from build123d import *

# Parameters (mm, degrees)
SKETCH1_W           = 12
SKETCH1_H           = 20
BOSS_EXTRUDE1_DEPTH = 2
SKETCH2_W           = 15
SKETCH2_H           = 4
BOSS_EXTRUDE2_DEPTH = 70


with BuildPart() as part:
    # Sketch1 → Boss-Extrude1 (new body)
    with BuildSketch(Plane(origin=(0, 0, 0), x_dir=(1, 0, 0), z_dir=(0, 1, 0))):
        with Locations((6, 20)):
            Rectangle(SKETCH1_W, SKETCH1_H)
        Polygon((102.5, 0), (110, 0), (110, 10), (12, 10), (0, 10), (0, 0), align=None)
        Polygon((117.5, 0), (110, 0), (102.5, 0), (102.5, -5), (117.5, -5), align=None)
        Polygon((110, 10), (110, 0), (117.5, 0), (220, 0), (220, 10), (208, 10), align=None)
        with Locations((214, 20)):
            Rectangle(SKETCH1_W, SKETCH1_H)
    extrude(amount=BOSS_EXTRUDE1_DEPTH)

    # Sketch2 → Boss-Extrude2 (add)
    with BuildSketch(Plane.XZ):
        with Locations((110, 3)):
            Rectangle(SKETCH2_W, SKETCH2_H)
    extrude(amount=BOSS_EXTRUDE2_DEPTH)


solid = part.part
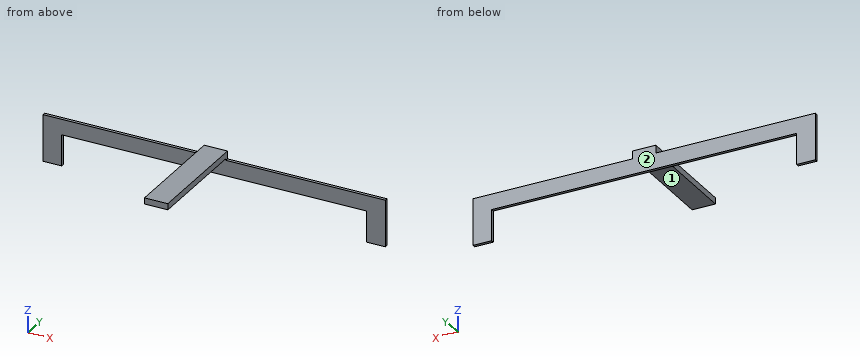
The listing builds one solid part. Answer for the finished solid, in the listing's coordinates (mm). Face numbers are marked on the shaded views. A direction names the side the tool comes from. Give positions to 0.01 mm unless a question says otherwise; leave off trailing zeros. Order: outer loops, then holes, each group sorted by start corner. A loop starts at its lowest first (then second) coordinate and runs counter-clockwise, first axis right, second up. Notation, with made-up numbers: (51.25, 70) - (84.25, 70) arc R25 ccw to (84.25, 107) - close; hole circle Ø11 at (80, -20). An arc over 180 degrees is marked (long way). One line per item, written item: value. Start each with the question number.
1) A cutting plane is placed at C-C on y = -54.5. Give the vertices of the cut face in (x, z), then the cut area to 3 significant figures.
2) A tool of negligible diameter and unlimited length cuts with its end or side. For the marked faces 1 and 2, from which of +Z, -Z, +X, -X, +Y, -Y can it reach the whole face along a straight path? Write none if from no direction.
3) A cutting plane is placed at B-B on x = 114. Give the vertices of the cut face in (y, z).
4) A cutting plane is placed at D-D on z = -4.5. Give the vertices of the cut face in (x, y).
5) Find the intervals of material crossed by L1, parallel to Y at x = 27.5, z = -7; L2, parallel to Z at x = 115, y = -66, in increasing order.
6) A cutting plane is placed at A-A on z = -19.5. Give the vertices of the cut face in (x, y).
7) Given pin 1 Ø0.6 at (x, y) = (43, 1.5) entering from +Z; pin 2 Ø2 at (y, z) = (0.5, -19.5) entering from -X; pin 3 Ø16.5 at (x, y) = (113, -43) entering from -Z; pin 4 Ø1.5 at (y, z) = (-47.5, 2) entering from +X, each flat-ended and moving along its own axis, determine where each tip first touches the part or whether it passes through.
Answer sheet:
1. outline: (102.5, 1) - (117.5, 1) - (117.5, 5) - (102.5, 5) - close
1. area: 60.0 mm2
2. face 1: -Z, +X, -X, -Y
2. face 2: +Z, -Z, +X, -X, +Y
3. outline: (-70, 1) - (0, 1) - (0, -10) - (2, -10) - (2, 5) - (-70, 5) - close
4. outline: (0, 0) - (220, 0) - (220, 2) - (0, 2) - close
5. L1: y = 0 to 2
5. L2: z = 1 to 5
6. outline: (0, 0) - (12, 0) - (12, 2) - (0, 2) - close; (208, 0) - (220, 0) - (220, 2) - (208, 2) - close
7. pin 1: stops at z = 0
7. pin 2: stops at x = 0
7. pin 3: stops at z = 1
7. pin 4: stops at x = 117.5
